from build123d import *

# Parameters (mm, degrees)
SKETCH2_R                         = 3.5
SKETCH2_R_2                       = 8
BOSS_EXTRUDE1_DEPTH               = 10
SKETCH4_R                         = 6
CUT_EXTRUDE1_DEPTH                = 6
CUT_EXTRUDE2_DEPTH                = 4
SKETCH6_R                         = 12.5
CUT_EXTRUDE3_DEPTH                = 10
TAP_DRILL_FOR_M10X1_25_TAP1_D     = 8.8
TAP_DRILL_FOR_M10X1_25_TAP1_DEPTH = 24
TAP_DRILL_FOR_M10X1_25_TAP1_TIP   = 2.643786724


with BuildPart() as part:
    # Sketch2 → Boss-Extrude1 (new, symmetric)
    with BuildSketch(Plane.XY):
        with BuildLine():
            Line((-46, 0), (-46, -125))
            Line((-46, -125), (46, -125))
            Line((46, -125), (46, 0))
            ThreePointArc((46, 0), (0, 46), (-46, 0))
        make_face()
        with Locations((0, 36)):
            Circle(SKETCH2_R, mode=Mode.SUBTRACT)
        Circle(SKETCH2_R_2, mode=Mode.SUBTRACT)
        with Locations((31.176914536, 18)):
            Circle(SKETCH2_R, mode=Mode.SUBTRACT)
        with Locations((31.176914536, -18)):
            Circle(SKETCH2_R, mode=Mode.SUBTRACT)
        with Locations((0, -36)):
            Circle(SKETCH2_R, mode=Mode.SUBTRACT)
        with Locations((-31.176914536, -18)):
            Circle(SKETCH2_R, mode=Mode.SUBTRACT)
        with Locations((-31.176914536, 18)):
            Circle(SKETCH2_R, mode=Mode.SUBTRACT)
    extrude(amount=BOSS_EXTRUDE1_DEPTH, both=True)

    # Sketch4 → Cut-Extrude1 (cut)
    with BuildSketch(Plane.XY.offset(10)):
        with Locations((0, 36)):
            Circle(SKETCH4_R)
        with Locations((31.176914536, 18)):
            Circle(SKETCH4_R)
        with Locations((31.176914536, -18)):
            Circle(SKETCH4_R)
        with Locations((0, -36)):
            Circle(SKETCH4_R)
        with Locations((-31.176914536, -18)):
            Circle(SKETCH4_R)
        with Locations((-31.176914536, 18)):
            Circle(SKETCH4_R)
    extrude(amount=-CUT_EXTRUDE1_DEPTH, mode=Mode.SUBTRACT)

    # Sketch5 → Cut-Extrude2 (cut)
    with BuildSketch(Plane.XY.offset(10)):
        with BuildLine():
            Line((34, -107), (34, -50.793700397))
            ThreePointArc((34, -50.793700397), (31.051285766, -45.627497229), (25.103448276, -45.539179666))
            ThreePointArc((25.103448276, -45.539179666), (0, -52), (-25.103448276, -45.539179666))
            ThreePointArc((-25.103448276, -45.539179666), (-31.051285766, -45.627497229), (-34, -50.793700397))
            Line((-34, -50.793700397), (-34, -107))
            ThreePointArc((-34, -107), (-32.242640687, -111.242640687), (-28, -113))
            Line((-28, -113), (28, -113))
            ThreePointArc((28, -113), (32.242640687, -111.242640687), (34, -107))
        make_face()
    cut_extrude2 = extrude(amount=-CUT_EXTRUDE2_DEPTH, mode=Mode.SUBTRACT)

    # Mirror1: Cut-Extrude2 across plane
    add(cut_extrude2.mirror(Plane.XY), mode=Mode.SUBTRACT)

    # Sketch6 → Cut-Extrude3 (cut)
    with BuildSketch(Plane(origin=(0, 0, -10), x_dir=(-1, 0, 0), z_dir=(0, 0, -1))):
        Circle(SKETCH6_R)
    extrude(amount=-CUT_EXTRUDE3_DEPTH, mode=Mode.SUBTRACT)

    # Tap Drill for M10x1.25 Tap1
    with Locations(Plane(origin=(0, -125, 0), x_dir=(-1, 0, 0), z_dir=(0, -1, 0))):
        with Locations((-30, 0), (30, 0)):
            Hole(TAP_DRILL_FOR_M10X1_25_TAP1_D / 2, depth=TAP_DRILL_FOR_M10X1_25_TAP1_DEPTH)
            with Locations((0, 0, -(TAP_DRILL_FOR_M10X1_25_TAP1_DEPTH + TAP_DRILL_FOR_M10X1_25_TAP1_TIP / 2))):  # 118° drill point
                Cone(0, TAP_DRILL_FOR_M10X1_25_TAP1_D / 2, TAP_DRILL_FOR_M10X1_25_TAP1_TIP, mode=Mode.SUBTRACT)


solid = part.part
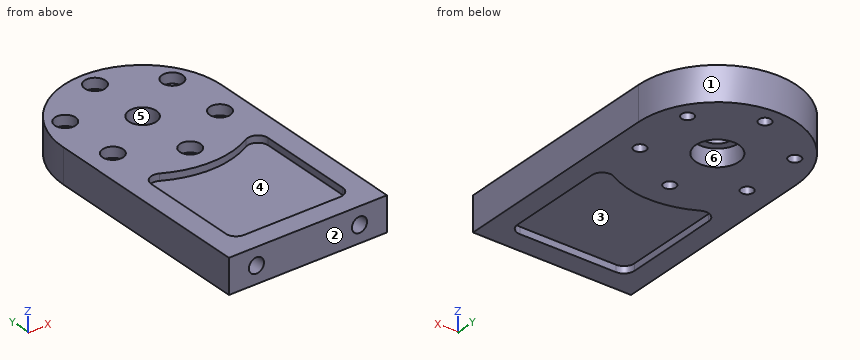
Source: CAD feature listing. Evaluate the final solid. Frame: model axes, mm. Face numbers are marked on the shaded views. A direction names the side the tool comes from. Give positions to 0.01 mm unless a question says otherwise; leave off trailing zeros. Write each loop counter-clockwise with the first axis right and the second up, starting at its lowest first coordinate (ties: lowest second). Pieces come first, ordered by that corner, then holes. Notation, with made-up numbers: M 42.5,77.25 L 99.5,77.25 A30 ccw 99.5,115.25 Z; hole C 63,27 d5. An arc over 180 degrees is marked long. Return JSON: item names as keys, results as strings. Group by question number.
1) Draft query along X for the marked faces 1, 2 and 3. Return one class per face: released by +X, released by -X, zero draft, split by the parting line, or undercut.
2) Cut plane D-D, the plane x = -15. Output: boundary loops of the cut face in (y, z).
3) First-contact query: pin 1 Ø11 at (x, y) = (31.18, 18) entering from -Z; pin 2 Ø6 at (y, z) = (13, -4.5) entering from +X; pin 3 Ø4.5 at (x, z) = (5.5, 9) entering from +Y; pin 4 Ø3 at (y, z) = (9, -4) entering from +X. Flat tips, straight axial feed; report the tip coordinate or a pass-through.
4) Cut plane B-B, the plane y = -36. Output: boundary loops of the cut face in (x, z), then the cut area to 3 significant figures.
5) Cut plane A-A, the plane z = -8. Give the number of separate pieces and of enclosed holes in the cut face, then the cut area to 3 significant figures.
6) Cut plane C-C, the plane y = -62.5. Output: boundary loops of the cut face in (x, z), then the cut area to 3 significant figures.
7) Ray query, L1, parallel to Y at x = 0, z = 6.5; L2, parallel to Y at x = 0, z = -1; L3, parallel to X at y = 23.5, z = 6.25. Return the intervals inside material, ascending.
8) Set-up query: the marked faces 4, 5 and 6. Return all of +Z, -Z, +X, -X, +Y, -Y with unobstructed straight access to the full face (end or side cutting, diameter ignored); none if empty.
Data:
{
 "1": {"face 1": "split by the parting line", "face 2": "zero draft", "face 3": "undercut"},
 "2": {"outline": "M -125,-10 L -113,-10 L -113,-6 L -49.79,-6 L -49.79,-10 L 43.49,-10 L 43.49,10 L -49.79,10 L -49.79,6 L -113,6 L -113,10 L -125,10 Z"},
 "3": {"pin 1": "stops at z = -10", "pin 2": "stops at x = 44.9", "pin 3": "stops at y = 45.89", "pin 4": "stops at x = 45.38"},
 "4": {"outline": "M -46,-10 L -3.5,-10 L -3.5,4 L -6,4 L -6,10 L -46,10 Z; M 3.5,-10 L 46,-10 L 46,10 L 6,10 L 6,4 L 3.5,4 Z", "area": "1,670 mm²"},
 "5": {"separate pieces": "1", "enclosed holes": "8", "area": "9,750 mm²"},
 "6": {"outline": "M -46,-10 L -34,-10 L -34,-6 L 34,-6 L 34,-10 L 46,-10 L 46,10 L 34,10 L 34,6 L -34,6 L -34,10 L -46,10 Z", "area": "1,300 mm²"},
 "7": {"L1": "y = -125 to -113, -52 to -42, -30 to -8, 8 to 30, 42 to 46", "L2": "y = -125 to -39.5, -32.5 to -12.5, 12.5 to 32.5, 39.5 to 46", "L3": "x = -39.54 to -33.57, -28.78 to 28.78, 33.57 to 39.54"},
 "8": {"face 4": "+Z", "face 5": "+Z, -Z", "face 6": "-Z"}
}
